Check sheet for the modelled part. Datum: model origin and axes. Units: mm. Round coordinates to 2 decimals unless told otherwise and drop trailing zeros. Write each loop counter-clockwise with the first axis right and the second up, starting at its lowest first coordinate (ties: lowest second). Pieces come first, ordered by that corner, then holes. Notation, with made-up numbers: (0.5, 65) - (25.5, 65) arc R14 ccw to (25.5, 82) - close; hole circle Ø11 at (-9, -40). An arc over 180 degrees is marked (long way). Answer as a JSON object with one key per item and string values. Group by question number.
Item 1: Gauge pin test, flat end, axial feed: P1, Ø10, axis at x = -254, z = 6.35, coming from the +Y side. Record the tip position at first contact, or that the pin passes through.
Item 2: Sectioned sample at A-A on z = 18.5. Record the boundary of the cut face in (x, y), plus the area to 3 significant figures.
Item 3: Thickness scan on line 1 (X direction, y = 1.05, z = 16); line 2 (Z direction, x = 0, y = -0.3) (3 decimals). Record the ranges inside material, lowest first.
Item 4: Sectioned sample at B-B on y = -0.6. Count the separate pieces of the cut face and the enclosed holes in it, plus the area to 3 significant figures.
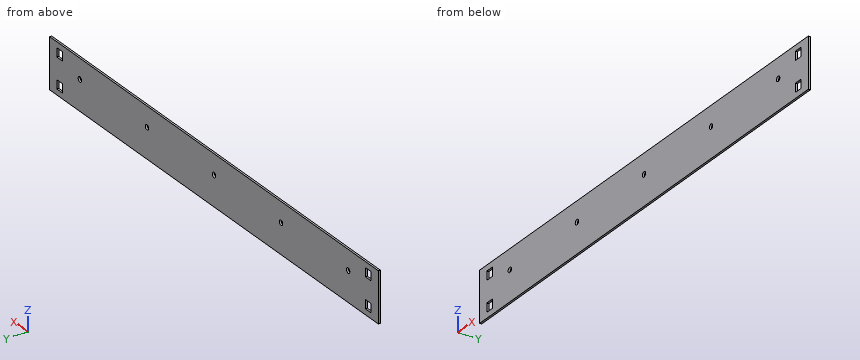
```python
from build123d import *

# Parameters (mm, degrees)
F0_W     = 622.3
F0_H     = 63.5
F0_W_2   = 11.1125
F0_H_2   = 11.1125
F0_R     = 3.175
F1_DEPTH = 1.27


with BuildPart() as f1:
    # F0 (on Front) → F1 (new body, symmetric)
    with BuildSketch(Plane.XZ):
        Rectangle(F0_W, F0_H)
        with Locations((-292.1, -19.05)):
            Rectangle(F0_W_2, F0_H_2, mode=Mode.SUBTRACT)
        with Locations((292.1, -19.05)):
            Rectangle(F0_W_2, F0_H_2, mode=Mode.SUBTRACT)
        with Locations((-254, 6.35)):
            Circle(F0_R, mode=Mode.SUBTRACT)
        with Locations((-127, 6.35)):
            Circle(F0_R, mode=Mode.SUBTRACT)
        with Locations((-292.1, 19.05)):
            Rectangle(F0_W_2, F0_H_2, mode=Mode.SUBTRACT)
        with Locations((0, 6.35)):
            Circle(F0_R, mode=Mode.SUBTRACT)
        with Locations((127, 6.35)):
            Circle(F0_R, mode=Mode.SUBTRACT)
        with Locations((254, 6.35)):
            Circle(F0_R, mode=Mode.SUBTRACT)
        with Locations((292.1, 19.05)):
            Rectangle(F0_W_2, F0_H_2, mode=Mode.SUBTRACT)
    extrude(amount=F1_DEPTH, both=True)


solid = f1.part
```
Completed:
{
 "1": {"P1": "y = 1.27"},
 "2": {"outline": "(-311.15, -1.27) - (-297.66, -1.27) - (-297.66, 1.27) - (-311.15, 1.27) - close; (-286.54, -1.27) - (286.54, -1.27) - (286.54, 1.27) - (-286.54, 1.27) - close; (297.66, -1.27) - (311.15, -1.27) - (311.15, 1.27) - (297.66, 1.27) - close", "area": "1,520 mm²"},
 "3": {"line 1": "-311.15 to -297.66, -286.54 to 286.54, 297.66 to 311.15", "line 2": "-31.75 to 3.175, 9.525 to 31.75"},
 "4": {"separate pieces": "1", "enclosed holes": "9", "area": "38,900 mm²"}
}
